```python
from build123d import *

# Parameters (mm, degrees)
F0_W     = 67.1
F0_H     = 138.3
F1_DEPTH = 7.2
F2_R     = 4.27
F3_DEPTH = 1
F4_R     = 9.08
F5_R     = 3.55


with BuildPart() as f1:
    # F0 (on Front) → F1 (new body)
    with BuildSketch(Plane.XZ):
        with Locations((0, 69.15)):
            Rectangle(F0_W, F0_H)
    extrude(amount=F1_DEPTH)

    # F2 (on face) → F3 (join)
    with BuildSketch(Plane.XZ.offset(7.2)):
        with Locations((-23.18, 128.13)):
            Circle(F2_R)
    extrude(amount=F3_DEPTH)

    # F4
    f4_edges = [f1.edges().sort_by_distance(p)[0] for p in [
        (-33.55, -3.6, 138.3),
        (33.55, -3.6, 138.3),
        (33.55, -3.6, 0),
        (-33.55, -3.6, 0),
    ]]
    fillet(f4_edges, radius=F4_R)

    # F5
    f5_edges = [f1.edges().sort_by_distance(p)[0] for p in [
        (0, -7.2, 138.3),
        (0, 0, 138.3),
    ]]
    fillet(f5_edges, radius=F5_R)


solid = f1.part
```
Could you check a few things on this model? Use its own coordinates, in mm. A direction names the side the tool comes from. Round coordinates to 2 decimals unless told otherwise and drop trailing zeros. Loops run counter-clockwise (first coordinate to the right, second up) from the corner with the lowest first, then second, coordinate; pieces in that order, holes last. Notation, with made-up numbers: (35, 22.25) - (84, 22.25) arc R13 ccw to (84, 45.25) - close; hole circle Ø2 at (87, 13). An arc over 180 degrees is marked (long way). Answer in a Markdown table with one row per item. Add a question column.
(1) I'm going to push flat-ended pins straight in: pin 1 (4 mm diameter, centred on x = 26, z = 36, fed in from -Y); pin 2 (1.5 mm diameter, centred on y = -2.5, z = 115, fed in from -X). Where does each tip first touch, or does it pass through?
(2) For faces 1 (the face through (-19, -8, 129)), 2 (the face through (32.48, -6.19, 68.31)), which set-ups out of +Z, -Z, +X, -X, +Y, -Y let a thin tool reach every point of the face, with its end or its side?
(3) If we section it at A-A (x = 19): Please give me the cut outline in (y, z), plus the area to 3 significant figures.
(4) If we section it at B-B (z = 16.5): Please give me the cut outline in (x, y), plus the area to 3 significant figures.
(5) I need wall thicknesses on line 1 along Y through (x, z) = (9.5, 43); line 2 along Z through (x, y) = (5, -4); line 3 along Z through (x, y) = (-13, -5.25). Which ranges of each line are inside material? Lowest first, please.
(6) If we section it at C-C (x = -23.18): Please give me the cut outline in (y, z), plus the area to 3 significant figures.
Model answer:
| question | item | result |
|---|---|---|
| 1 | pin 1 | stops at y = -7.2 |
| 1 | pin 2 | stops at x = -33.54 |
| 2 | face 1 | -Y |
| 2 | face 2 | +Z, -Z, +X, -Y |
| 3 | outline | (-7.2, 3.55) arc R3.55 ccw to (-3.65, 0) - (-3.55, 0) arc R3.55 ccw to (0, 3.55) - (0, 134.75) arc R3.55 ccw to (-3.55, 138.3) - (-3.65, 138.3) arc R3.55 ccw to (-7.2, 134.75) - close |
| 3 | area | 985 mm² |
| 4 | outline | (-33.55, -3.65) arc R3.55 ccw to (-30, -7.2) - (30, -7.2) arc R3.55 ccw to (33.55, -3.65) - (33.55, -3.55) arc R3.55 ccw to (30, 0) - (-30, 0) arc R3.55 ccw to (-33.55, -3.55) - close |
| 4 | area | 472 mm² |
| 5 | line 1 | y = -7.2 to 0 |
| 5 | line 2 | z = 0.02 to 138.28 |
| 5 | line 3 | z = 0.38 to 137.92 |
| 6 | outline | (-8.2, 123.86) - (-7.2, 123.86) - (-7.2, 3.55) arc R3.55 ccw to (-3.65, 0) - (-3.55, 0) arc R3.55 ccw to (0, 3.55) - (0, 134.75) arc R3.55 ccw to (-3.55, 138.3) - (-3.65, 138.3) arc R3.55 ccw to (-7.2, 134.75) - (-7.2, 132.4) - (-8.2, 132.4) - close |
| 6 | area | 993 mm² |
